```python
from build123d import *

# Parameters (mm, degrees)
F0_R     = 25.4
F1_DEPTH = 6.35
F2_R     = 22.225
F3_DEPTH = 12.7
F4_R     = 25.4
F5_DEPTH = 6.35
F6_R     = 1.6002
F7_R     = 6.35
F7_R_2   = 1.5875
F8_DEPTH = 3.175


with BuildPart() as f1:
    # F0 (on Front) → F1 (new body)
    with BuildSketch(Plane.XZ):
        Circle(F0_R)
    extrude(amount=F1_DEPTH)

    # F2 (on face) → F3 (join)
    with BuildSketch(Plane.XZ.offset(6.35)):
        Circle(F2_R)
    extrude(amount=F3_DEPTH)

    # F4 (on face) → F5 (join)
    with BuildSketch(Plane.XZ.offset(19.05)):
        Circle(F4_R)
    extrude(amount=F5_DEPTH)

    # F6
    f6_edges = [f1.edges().sort_by_distance(p)[0] for p in [
        (25.4, -3.175, 0),
        (-25.4, 0, 0),
        (-25.4, -6.35, 0),
        (25.4, -22.225, 0),
        (-25.4, -19.05, 0),
        (-25.4, -25.4, 0),
    ]]
    fillet(f6_edges, radius=F6_R)

    # F7 (on face) → F8 (cut)
    with BuildSketch(Plane.XZ.offset(25.4)):
        Circle(F7_R)
        with Locations((0, 19.05)):
            Circle(F7_R_2)
        with Locations((19.05, 0)):
            Circle(F7_R_2)
        with Locations((0, -19.05)):
            Circle(F7_R_2)
        with Locations((-19.05, 0)):
            Circle(F7_R_2)
    extrude(amount=-F8_DEPTH, mode=Mode.SUBTRACT)


solid = f1.part
```
Work out the finished part from the listing and answer in its coordinate system (mm). A direction names the side the tool comes from. Give positions to 0.01 mm unless a question says otherwise; leave off trailing zeros. Write each loop counter-clockwise with the first axis right and the second up, starting at its lowest first coordinate (ties: lowest second). Pieces come first, ordered by that corner, then holes.
(1) Straight lines are drawn through the part: line 1 (Y direction, x = -17.5, z = -15); line 2 (Y direction, x = 21, z = 13.5); line 3 (X direction, y = -22.75, z = 5). For each, find the intervals that lie inside material, in ascending order.
Final values:
line 1: y = -25.4 to -19.05, -6.35 to 0
line 2: y = -24.9 to -19.55, -5.85 to -0.5
line 3: x = -24.9 to -3.91, 3.91 to 24.9
(2) The part is cut by section C-C on y = -14.25. Write down the section's boundary in (x, z) (3 decimals), plus the area to 3 significant figures.
Final values:
outline: circle Ø44.45 at (0, 0)
area: 1,550 mm2
(3) The mould has two halves that part along X. Classify faces 1 (the cylindrical face through (-5.506, -3.153, -24.796)), 2 (the flat face through (0, 0, 0)), 3 (the flat face through (19, -22.225, 0)): pulls with the +X half, pulls with the -X half, needs draft (parallel to the pull), parting line crosses it, or undercut.
Final values:
face 1: parting line crosses it
face 2: needs draft
face 3: undercut
(4) Flat-ended cylindrical pins translate along their axes: pin 1 Ø1.5 at (x, y) = (14, -14.5) entering from -Z; pin 2 Ø3 at (y, z) = (-17, -9.5) entering from +X; pin 3 Ø1.9 at (x, z) = (19.05, 0) entering from -Y (3 decimals). Find the tip coordinate at first contact, or state that the pin passes through.
Final values:
pin 1: stops at z = -17.84
pin 2: stops at x = 20.74
pin 3: stops at y = -22.225
(5) Which of the six approach directions +Z, -Z, +X, -X, +Y, -Y give full straight-line access (tool end or side, diameter ignored) to faces 4 (the flat face through (5, -25.4, -5)), 5 (the flat face through (-20, -6.35, 11)), 6 (the flat face through (-19, -22.225, 0))?
Final values:
face 4: +Z, -Z, +X, -X, -Y
face 5: none
face 6: -Y
(6) The part is cut by section D-D on y = -5.5. Write down the section's boundary in (x, z), plus the area to 3 significant figures.
Final values:
outline: circle Ø50.43 at (0, 0)
area: 2,000 mm2
